```python
from build123d import *

# Parameters (mm, degrees)
SKETCH_W     = 33
SKETCH_H     = 17
SKETCH_R     = 2.25
PAD_DEPTH    = 6.5
SKETCH001_R  = 3.75
POCKET_DEPTH = 2.5
FILLET_R     = 1.5


with BuildPart() as part:
    # Sketch → Pad (new body)
    with BuildSketch(Plane.XY):
        with Locations((16.5, 8.5)):
            Rectangle(SKETCH_W, SKETCH_H)
        with Locations((6.5, 8.5)):
            Circle(SKETCH_R, mode=Mode.SUBTRACT)
        with Locations((26.5, 8.5)):
            Circle(SKETCH_R, mode=Mode.SUBTRACT)
    extrude(amount=PAD_DEPTH)

    # Sketch001 (on Face8 of Pad) → Pocket (cut)
    with BuildSketch(Plane.XY.offset(6.5)):
        with Locations((6.5, 8.5)):
            Circle(SKETCH001_R)
        with Locations((26.5, 8.5)):
            Circle(SKETCH001_R)
    extrude(amount=-POCKET_DEPTH, mode=Mode.SUBTRACT)

    # Fillet
    fillet_edges = [part.edges().sort_by_distance(p)[0] for p in [
        (33, 8.5, 6.5),
        (0, 8.5, 6.5),
    ]]
    fillet(fillet_edges, radius=FILLET_R)


solid = part.part
```
Check sheet for the modelled part. Datum: model origin and axes. Units: mm. A direction names the side the tool comes from. Round coordinates to 2 decimals unless told otherwise and drop trailing zeros. Loops run counter-clockwise (first coordinate to the right, second up) from the corner with the lowest first, then second, coordinate; pieces in that order, holes last. Notation, with made-up numbers: (14, -30) -> (43, -30) arc R18 cw to (43, -3) -> close; hole circle Ø2 at (-6, 84.5). An arc over 180 degrees is marked (long way). Write item = value, one per line. Start each with the question number.
1) Gauge pin test, flat ends, axial feed: pin 1 Ø2.5 at (x, y) = (6.5, 8.5) entering from +Z; pin 2 Ø4 at (x, y) = (27, 7.5) entering from +Z; pin 3 Ø10 at (x, y) = (8.5, 8.5) entering from +Z. Record the tip position at first contact, or that the pin passes through.
2) Sectioned sample at C-C, the plane z = 5.5. Record the cut outline in (x, y).
3) Thickness scan on probe 1 along X at (y, z) = (8.5, 1.55); probe 2 along Y at (x, z) = (6.5, 1.3); probe 3 along Y at (x, z) = (6.5, 4.7). Record the ranges inside material, lowest first.
4) Sectioned sample at D-D, the plane x = 7.5. Record the cut outline in (y, z).
5) Sectioned sample at B-B, the plane y = 8.5. Record the cut outline in (x, z), plus the area to 3 significant figures.
6) Set-up check for faces 1 (the flat face through (0, 8, 2)), 2 (the flat face through (26, 6, 4)): record each of +Z, -Z, +X, -X, +Y, -Y from which the full face is reachable in a straight line by a thin tool's end or side.
7) Sectioned sample at A-A, the plane x = 26.5. Record the cut outline in (y, z).
8) Release check for a two-part mould opening along Y. For faces 3 (the cylindrical face through (27.71, 10.397, 1.972)), 4 (the flat face through (16, 0, 3)), 5 (the flat face through (16, 17, 3)), 6 (the flat face through (33, 8, 2)) record: released by +Y, released by -Y, zero draft, split by the parting line, or undercut.
Results are:
q1.pin_1 = through
q1.pin_2 = 4
q1.pin_3 = 6.5
q2.outline = (0.09, 0) -> (32.91, 0) -> (32.91, 17) -> (0.09, 17) -> close; hole circle Ø7.5 at (6.5, 8.5); hole circle Ø7.5 at (26.5, 8.5)
q3.probe_1 = 0 to 4.25, 8.75 to 24.25, 28.75 to 33
q3.probe_2 = 0 to 6.25, 10.75 to 17
q3.probe_3 = 0 to 4.75, 12.25 to 17
q4.outline = (0, 0) -> (6.48, 0) -> (6.48, 4) -> (4.89, 4) -> (4.89, 6.5) -> (0, 6.5) -> close; (10.52, 0) -> (17, 0) -> (17, 6.5) -> (12.11, 6.5) -> (12.11, 4) -> (10.52, 4) -> close
q5.outline = (0, 0) -> (4.25, 0) -> (4.25, 4) -> (2.75, 4) -> (2.75, 6.5) -> (1.5, 6.5) arc R1.5 ccw to (0, 5) -> close; (8.75, 0) -> (24.25, 0) -> (24.25, 4) -> (22.75, 4) -> (22.75, 6.5) -> (10.25, 6.5) -> (10.25, 4) -> (8.75, 4) -> close; (28.75, 0) -> (33, 0) -> (33, 5) arc R1.5 ccw to (31.5, 6.5) -> (30.25, 6.5) -> (30.25, 4) -> (28.75, 4) -> close
q5.area = 140 mm^2
q6.face_1 = +Z, -Z, -X, +Y, -Y
q6.face_2 = +Z
q7.outline = (0, 0) -> (6.25, 0) -> (6.25, 4) -> (4.75, 4) -> (4.75, 6.5) -> (0, 6.5) -> close; (10.75, 0) -> (17, 0) -> (17, 6.5) -> (12.25, 6.5) -> (12.25, 4) -> (10.75, 4) -> close
q8.face_3 = undercut
q8.face_4 = released by -Y
q8.face_5 = released by +Y
q8.face_6 = zero draft
